Design review of the part built by this model. Coordinates are the model's own, in mm. Face numbers are marked on the shaded views. A direction names the side the tool comes from. Coordinates: 2 decimals unless noted, no trailing zeros. Write each loop counter-clockwise with the first axis right and the second up, starting at its lowest first coordinate (ties: lowest second). Pieces come first, ordered by that corner, then holes.
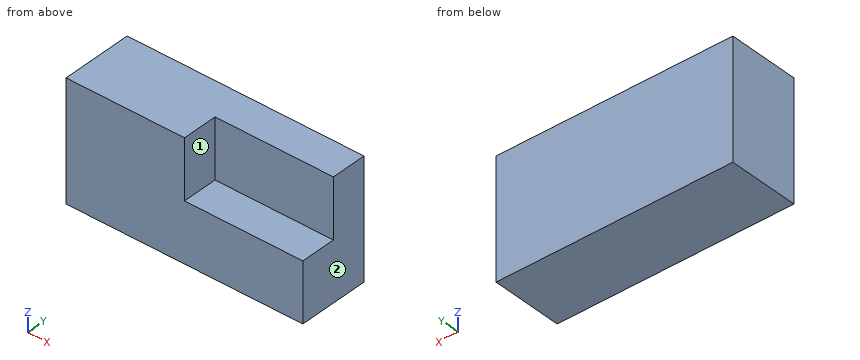
```python
from build123d import *

# Parameters (mm, degrees)
F1_DEPTH = 38.1
F0_W     = 63.5
F0_H     = 31.75
F2_DEPTH = 19.05


with BuildPart() as f1:
    # F0 (on Front) → F1 (new body)
    with BuildSketch(Plane.XZ):
        Polygon((-67.157373, 0), (-67.157373, -63.5), (59.842627, -63.5), (59.842627, -31.75), (-3.657373, -31.75), (-3.657373, 0), align=None)
    extrude(amount=F1_DEPTH)

    # F0 (on Front) → F2 (join)
    with BuildSketch(Plane.XZ):
        Polygon((-67.157373, 0), (-67.157373, -63.5), (59.842627, -63.5), (59.842627, -31.75), (-3.657373, -31.75), (-3.657373, 0), align=None)
        with Locations((28.092627, -15.875)):
            Rectangle(F0_W, F0_H)
    extrude(amount=F2_DEPTH)


solid = f1.part
```
(1) Consider section A-A (z = -25). Give the boundary of the cut face in (x, y).
(2) Consider section B-B (x = 35.5). Give the boundary of the cut face in (y, z).
(3) Wall thickness on line 1 (X direction, y = -28.5, z = -18); line 2 (Z direction, x = -3.5, y = -29.5); line 3 (Y direction, x = 29.5, z = -11): over which ranges is each line inside the solid? List them lowest first.
(4) Insertion check: pin 1 Ø3 at (y, z) = (-21, -24.5) entering from +X; pin 2 Ø3 at (x, y) = (40, -30) entering from +Z; pin 3 Ø9.5 at (x, z) = (14, -20.5) entering from -Y. Each pin has a flat end and moves straight along its axis. Give the tip position at first contact, or say it passes through.
(5) For the marked faces 1 and 2, list the 3-axis set-ups (+Z, -Z, +X, -X, +Y, -Y) from which the entire face can be reached by the end or side of a thin tool; tool diameter is ignored.
Results:
1. outline: (-67.16, -38.1) - (-3.66, -38.1) - (-3.66, -19.05) - (59.84, -19.05) - (59.84, 0) - (-67.16, 0) - close
2. outline: (-38.1, -63.5) - (0, -63.5) - (0, 0) - (-19.05, 0) - (-19.05, -31.75) - (-38.1, -31.75) - close
3. line 1: x = -67.16 to -3.66
3. line 2: z = -63.5 to -31.75
3. line 3: y = -19.05 to 0
4. pin 1: stops at x = -3.66
4. pin 2: stops at z = -31.75
4. pin 3: stops at y = -19.05
5. face 1: +Z, +X, -Y
5. face 2: +Z, -Z, +X, +Y, -Y
